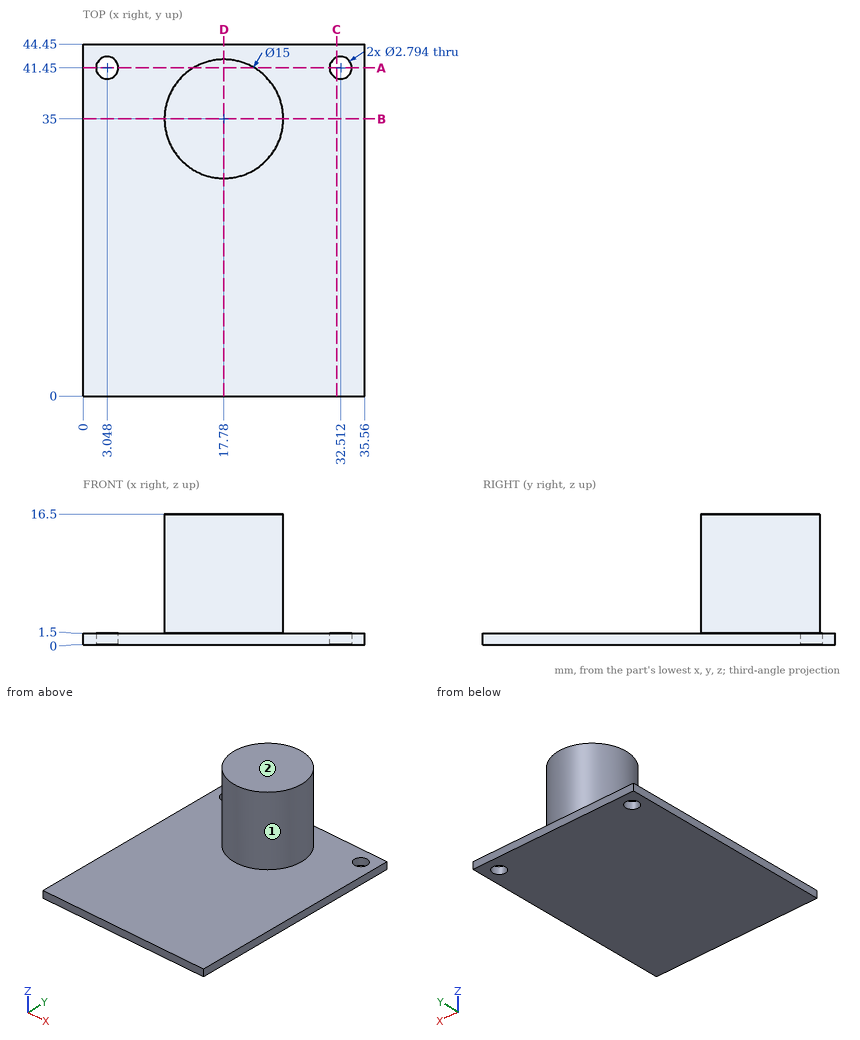
Can you work these out from the drawing? Everything is in mm from the part's minimum corner. A direction names the side the tool comes from. Coordinates: 2 decimals unless noted, no trailing zeros. Write each loop counter-clockwise with the first axis right and the second up, starting at its lowest first coordinate (ties: lowest second). Pieces come first, ordered by that corner, then holes. Notation, with made-up numbers: (3, 81) - (51, 81) arc R15 ccw to (51, 91) - close; hole circle Ø4 at (-37.75, -29). An arc over 180 degrees is marked (long way). Use a Markdown table: item, result.
Q1. Please list where these lines run through material, in increasing order: L1, parallel to Y at x = 18, z = 9.5; L2, parallel to Z at x = 23, y = 5; L3, parallel to Y at x = 11, z = 11.25.
Geometry check:
| item | result |
|---|---|
| L1 | y = 27.5 to 42.5 |
| L2 | z = 0 to 1.5 |
| L3 | y = 31.79 to 38.21 |
Q2. Imagine slicing it at D-D (x = 17.78). List the corners of the cut face in (y, z) for me, and give its area (3 significant figures).
Geometry check:
| item | result |
|---|---|
| outline | (0, 0) - (44.45, 0) - (44.45, 1.5) - (42.5, 1.5) - (42.5, 16.5) - (27.5, 16.5) - (27.5, 1.5) - (0, 1.5) - close |
| area | 292 mm2 |
Q3. Imagine slicing it at B-B (y = 35). List the corners of the cut face in (x, z) for me, and give its area (3 significant figures).
Geometry check:
| item | result |
|---|---|
| outline | (0, 0) - (35.56, 0) - (35.56, 1.5) - (25.28, 1.5) - (25.28, 16.5) - (10.28, 16.5) - (10.28, 1.5) - (0, 1.5) - close |
| area | 278 mm2 |
Q4. Which directions (+Z, -Z, +X, -X, +Y, -Y) give clear straight access to the entire face, cutting with the end or side of a thin tool? Please do the marked faces 1 and 2.
Geometry check:
| item | result |
|---|---|
| face 1 | +Z |
| face 2 | +Z, +X, -X, +Y, -Y |
Q5. Imagine slicing it at C-C (x = 32). List the corners of the cut face in (y, z) for me, and give its area (3 significant figures).
Geometry check:
| item | result |
|---|---|
| outline | (0, 0) - (40.15, 0) - (40.15, 1.5) - (0, 1.5) - close; (42.75, 0) - (44.45, 0) - (44.45, 1.5) - (42.75, 1.5) - close |
| area | 62.8 mm2 |
Q6. Imagine slicing it at A-A (y = 41.45). List the corners of the cut face in (x, z) for me (3 decimals).
Geometry check:
| item | result |
|---|---|
| outline | (0, 0) - (1.651, 0) - (1.651, 1.5) - (0, 1.5) - close; (4.445, 0) - (31.115, 0) - (31.115, 1.5) - (21.607, 1.5) - (21.607, 16.5) - (13.953, 16.5) - (13.953, 1.5) - (4.445, 1.5) - close; (33.909, 0) - (35.56, 0) - (35.56, 1.5) - (33.909, 1.5) - close |
Q7. I'm going to push flat-ended pins straight in: pin 1 Ø1.5 at (x, y) = (19.5, 9.5) entering from +Z; pin 2 Ø6 at (x, y) = (9.5, 18.5) entering from -Z. Where does each tip first touch, or does it pass through?
Geometry check:
| item | result |
|---|---|
| pin 1 | stops at z = 1.5 |
| pin 2 | stops at z = 0 |
